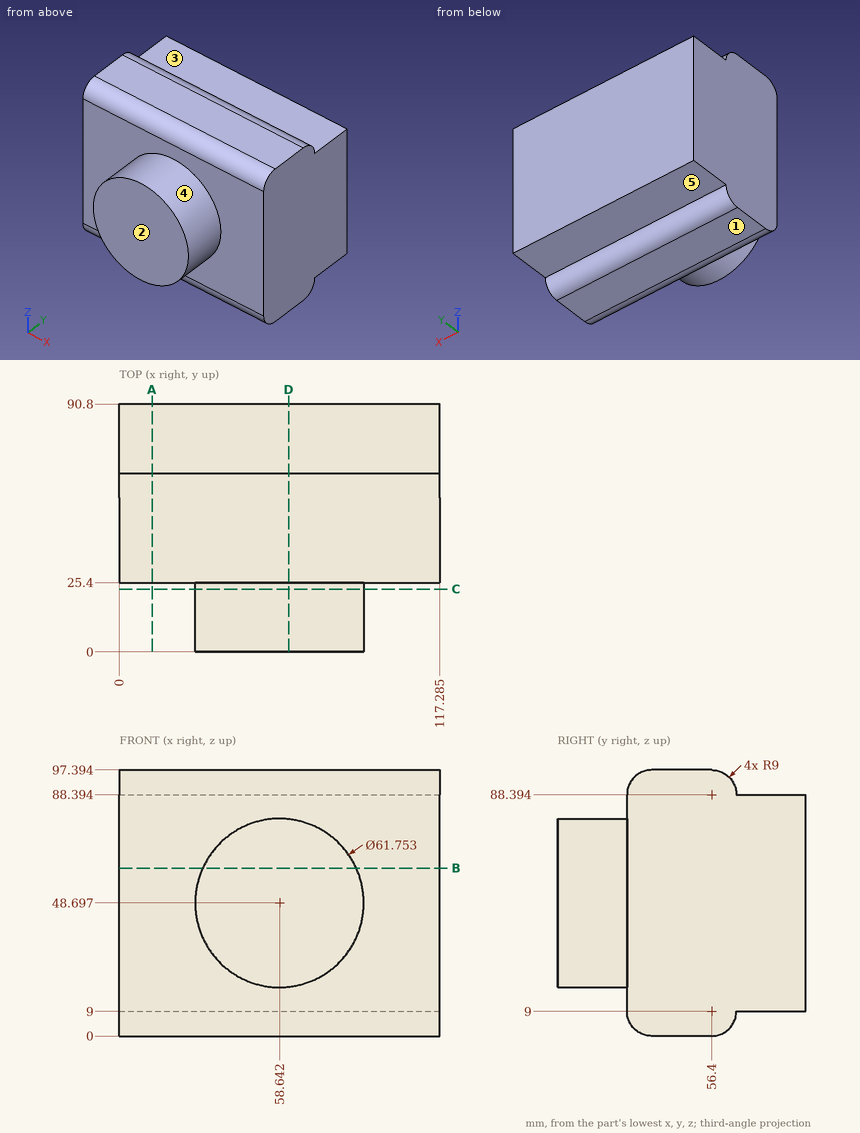
Geometry check sheet. Reference: drawing and pictorial views, mm from the part's lowest x, y, z. A direction names the side the tool comes from. Coordinates: 2 decimals unless noted, no trailing zeros. Loops run counter-clockwise (first coordinate to the right, second up) from the corner with the lowest first, then second, coordinate; pieces in that order, holes last. Notation, with made-up numbers: (59.5, -31) -> (67.5, -31) arc R25 ccw to (67.5, -4) -> close; hole circle Ø7 at (-4.5, 70.5). An arc over 180 degrees is marked (long way). Put each result on its own line as item: value.
1) Cross-section at A-A on x = 12. Record the boundary of the cut face in (y, z), plus the area to 3 significant figures.
Result set:
outline: (25.4, 9) arc R9 ccw to (34.4, 0) -> (56.4, 0) arc R9 ccw to (65.4, 9) -> (90.8, 9) -> (90.8, 88.39) -> (65.4, 88.39) arc R9 ccw to (56.4, 97.39) -> (34.4, 97.39) arc R9 ccw to (25.4, 88.39) -> close
area: 5,840 mm^2
2) Cross-section at C-C on y = 23. Record the boundary of the cut face in (x, z), plus the area to 4 significant figures.
Result set:
outline: circle Ø61.75 at (58.64, 48.7)
area: 2,995 mm^2
3) Cross-section at B-B on z = 61.5. Record the boundary of the cut face in (x, y) (1 decimal).
Result set:
outline: (0, 25.4) -> (30.5, 25.4) -> (30.5, 0) -> (86.7, 0) -> (86.7, 25.4) -> (117.3, 25.4) -> (117.3, 90.8) -> (0, 90.8) -> close
4) Cross-section at D-D on x = 62. Record the boundary of the cut face in (y, z), plus the area to 3 significant figures.
Result set:
outline: (0, 18) -> (25.4, 18) -> (25.4, 9) arc R9 ccw to (34.4, 0) -> (56.4, 0) arc R9 ccw to (65.4, 9) -> (90.8, 9) -> (90.8, 88.39) -> (65.4, 88.39) arc R9 ccw to (56.4, 97.39) -> (34.4, 97.39) arc R9 ccw to (25.4, 88.39) -> (25.4, 79.39) -> (0, 79.39) -> close
area: 7,400 mm^2
5) Gauge pin test, flat ends, axial feed: pin 1 Ø4 at (x, y) = (77.5, 18) entering from -Z; pin 2 Ø7.5 at (x, y) = (80.5, 73) entering from -Z; pin 3 Ø4 at (x, y) = (73, 24.5) entering from -Z; pin 4 Ø12 at (y, z) = (37.5, 29.5) entering from -X. Record the tip position at first contact, or that the pin passes through.
Result set:
pin 1: stops at z = 22.83
pin 2: stops at z = 9
pin 3: stops at z = 4.69
pin 4: stops at x = 0
6) Tool access check on the marked faces 1, 2, 3, 4 and 5. Record the directions out of +Z, -Z, +X, -X, +Y, -Y that give a thin tool (end or side, any length) a straight path to the whole face; none if there is none.
Result set:
face 1: -Z, +X, -X, +Y, -Y
face 2: +Z, -Z, +X, -X, -Y
face 3: +Z, +X, -X, +Y
face 4: -Y
face 5: -Z, +X, -X, +Y
7) Thickness scan on line 1 (Z direction, x = 89.5, y = 67.5); line 2 (Y direction, x = 32, z = 66); line 3 (Z direction, x = 58, y = 10). Record the ranges inside material, lowest first.
Result set:
line 1: z = 9 to 88.39
line 2: y = 25.4 to 90.8
line 3: z = 17.83 to 79.57
